```python
from build123d import *

# Parameters (mm, degrees)
SKETCH1_W                        = 100
SKETCH1_H                        = 85
BOSS_EXTRUDE1_DEPTH              = 105
SKETCH2_W                        = 71
SKETCH2_H                        = 91
CUT_EXTRUDE1_DEPTH               = 90
M10X1_0_TAPPED_HOLE1_D           = 9
M10X1_0_TAPPED_HOLE1_DEPTH       = 23
M10X1_0_TAPPED_HOLE1_CBORE_D     = 10
M10X1_0_TAPPED_HOLE1_CBORE_DEPTH = 20
M10X1_0_TAPPED_HOLE1_TIP         = 2.703872786
M10X1_0_TAPPED_HOLE2_D           = 9
M10X1_0_TAPPED_HOLE2_DEPTH       = 23
M10X1_0_TAPPED_HOLE2_CBORE_D     = 10
M10X1_0_TAPPED_HOLE2_CBORE_DEPTH = 20
M10X1_0_TAPPED_HOLE2_TIP         = 2.703872786
M10X1_0_TAPPED_HOLE3_D           = 9
M10X1_0_TAPPED_HOLE3_DEPTH       = 23
M10X1_0_TAPPED_HOLE3_CBORE_D     = 10
M10X1_0_TAPPED_HOLE3_CBORE_DEPTH = 20
M10X1_0_TAPPED_HOLE3_TIP         = 2.703872786


with BuildPart() as part:
    # Sketch1 → Boss-Extrude1 (new body)
    with BuildSketch(Plane(origin=(0, 0, 0), x_dir=(1, 0, 0), z_dir=(0, 1, 0))):
        with Locations((-11.958288623, 7.903366629)):
            Rectangle(SKETCH1_W, SKETCH1_H)
    extrude(amount=BOSS_EXTRUDE1_DEPTH)

    # Sketch2 → Cut-Extrude1 (cut)
    with BuildSketch(Plane(origin=(38.041711377, 0, 0), x_dir=(0, 0, -1), z_dir=(1, 0, 0))):
        with Locations((7.903366629, 52.5)):
            Rectangle(SKETCH2_W, SKETCH2_H)
    extrude(amount=-CUT_EXTRUDE1_DEPTH, mode=Mode.SUBTRACT)

    # M10x1.0 Tapped Hole1
    with Locations(Plane(origin=(-21.958288623, 85, 34.596633371), x_dir=(1, 0, 0), z_dir=(0, 0, 1))):
        with Locations((0, 0), (0, -60)):
            CounterBoreHole(M10X1_0_TAPPED_HOLE1_D / 2, M10X1_0_TAPPED_HOLE1_CBORE_D / 2, M10X1_0_TAPPED_HOLE1_CBORE_DEPTH, depth=M10X1_0_TAPPED_HOLE1_DEPTH)
            with Locations((0, 0, -(M10X1_0_TAPPED_HOLE1_DEPTH + M10X1_0_TAPPED_HOLE1_TIP / 2))):  # 118° drill point
                Cone(0, M10X1_0_TAPPED_HOLE1_D / 2, M10X1_0_TAPPED_HOLE1_TIP, mode=Mode.SUBTRACT)

    # M10x1.0 Tapped Hole2
    with Locations(Plane(origin=(-11.958288623, 0, -30.403366629), x_dir=(0, 0, -1), z_dir=(0, -1, 0))):
        with Locations((0, 0)):
            CounterBoreHole(M10X1_0_TAPPED_HOLE2_D / 2, M10X1_0_TAPPED_HOLE2_CBORE_D / 2, M10X1_0_TAPPED_HOLE2_CBORE_DEPTH, depth=M10X1_0_TAPPED_HOLE2_DEPTH)
            with Locations((0, 0, -(M10X1_0_TAPPED_HOLE2_DEPTH + M10X1_0_TAPPED_HOLE2_TIP / 2))):  # 118° drill point
                Cone(0, M10X1_0_TAPPED_HOLE2_D / 2, M10X1_0_TAPPED_HOLE2_TIP, mode=Mode.SUBTRACT)

    # M10x1.0 Tapped Hole3
    with Locations(Plane.ZY.offset(61.958288623)):
        with Locations((-7.903366629, 37.5), (-7.903366629, 52.5), (-7.903366629, 67.5)):
            CounterBoreHole(M10X1_0_TAPPED_HOLE3_D / 2, M10X1_0_TAPPED_HOLE3_CBORE_D / 2, M10X1_0_TAPPED_HOLE3_CBORE_DEPTH, depth=M10X1_0_TAPPED_HOLE3_DEPTH)
            with Locations((0, 0, -(M10X1_0_TAPPED_HOLE3_DEPTH + M10X1_0_TAPPED_HOLE3_TIP / 2))):  # 118° drill point
                Cone(0, M10X1_0_TAPPED_HOLE3_D / 2, M10X1_0_TAPPED_HOLE3_TIP, mode=Mode.SUBTRACT)


solid = part.part
```
Source: CAD feature listing. Evaluate the final solid. Frame: model axes, mm. A direction names the side the tool comes from. Give positions to 0.01 mm unless a question says otherwise; leave off trailing zeros. Loops run counter-clockwise (first coordinate to the right, second up) from the corner with the lowest first, then second, coordinate; pieces in that order, holes last. Notation, with made-up numbers: (20.25, -13.5) -> (73.25, -13.5) arc R12 ccw to (73.25, -8.5) -> close; hole circle Ø1 at (-17, 63). An arc over 180 degrees is marked (long way). Use a Markdown table: item, result. Add a question column.
(1) Section query B-B (x = 3). Output: boundary loops of the cut face in (y, z).
(2) Access query for faces 1 (the face through (-23.04, 20.12, 31.15)), 2 (the face through (-6, 98, -7)), 3 (the face through (-10.456, 3.451, -35.172)). Directions: +Z, -Z, +X, -X, +Y, -Y. A direction counts if a zero-diameter tool reaches every point of the face in a straight line with its end or side. Return the directions, or none.
(3) Section query D-D (y = 67.5). Output: boundary loops of the cut face in (x, z).
(4) First-contact query: pin 1 Ø21.5 at (y, z) = (41, 2) entering from +X. Flat tip, straight axial feed; report the tip coordinate or a pass-through.
(5) Section query A-A (y = 25). Output: boundary loops of the cut face in (x, z), then the cut area to 3 significant figures.
(6) Pull-direction query (Y, two-part tool) for faces 4 (the face through (-13, 0, -8)), 5 (the face through (-57.03, 41.72, -5.22)), 6 (the face through (38.042, 52, 30)); classes: +Y half, -Y half, draft (parallel to the pull), parting line (faces both ways), or undercut.
(7) Section query C-C (z = -20). Output: boundary loops of the cut face in (x, y), then the cut area to 3 significant figures.
(8) Ray query, line 1 (Y direction, x = 31.5, z = -5.5); line 2 (Z direction, x = -24.5, y = 66.5); line 3 (X direction, y = 30, z = -26). Return the intervals inside material, ascending.
Checked values:
| question | item | result |
|---|---|---|
| 1 | outline | (0, -50.4) -> (105, -50.4) -> (105, 34.6) -> (0, 34.6) -> close; hole (7, -43.4) -> (98, -43.4) -> (98, 27.6) -> (7, 27.6) -> close |
| 2 | face 1 | +Z |
| 2 | face 2 | +X |
| 2 | face 3 | -Y |
| 3 | outline | (-61.96, -50.4) -> (38.04, -50.4) -> (38.04, -43.4) -> (-51.96, -43.4) -> (-51.96, -12.9) -> (-61.96, -12.9) -> close; (-61.96, -2.9) -> (-51.96, -2.9) -> (-51.96, 27.6) -> (38.04, 27.6) -> (38.04, 34.6) -> (-61.96, 34.6) -> close |
| 4 | pin 1 | x = -51.96 |
| 5 | outline | (-61.96, -50.4) -> (38.04, -50.4) -> (38.04, -43.4) -> (-51.96, -43.4) -> (-51.96, 27.6) -> (-26.96, 27.6) -> (-26.96, 34.6) -> (-61.96, 34.6) -> close; (-16.96, 27.6) -> (38.04, 27.6) -> (38.04, 34.6) -> (-16.96, 34.6) -> close |
| 5 | area | 2,040 mm^2 |
| 6 | face 4 | -Y half |
| 6 | face 5 | undercut |
| 6 | face 6 | draft |
| 7 | outline | (-61.96, 0) -> (38.04, 0) -> (38.04, 7) -> (-51.96, 7) -> (-51.96, 98) -> (38.04, 98) -> (38.04, 105) -> (-61.96, 105) -> close |
| 7 | area | 2,310 mm^2 |
| 8 | line 1 | 0 to 7, 98 to 105 |
| 8 | line 2 | -50.4 to -43.4, 27.6 to 34.6 |
| 8 | line 3 | -61.96 to -51.96 |
